Check sheet for the drawn part. Datum: minimum x, y, z corner. Units: mm. Coordinates: 2 decimals unless noted, no trailing zeros. Order: outer loops, then holes, each group sorted by start corner. A loop starts at its lowest first (then second) coordinate and runs counter-clockwise, first axis right, second up.
Q1. Thickness scan on line 1 (X direction, y = 3.75, z = 20); line 2 (Y direction, x = 27.5, z = 24.5). Record the ranges inside material, lowest first.
Q2. Cross-section at A-A, the plane z = 20. Record the boundary of the cut face in (x, y).
Q3. Cross-section at B-B, the plane x = 20. Record the boundary of the cut face in (y, z).
Q4. Depth check by flat-ended pin: P1, Ø1.5, axis at x = 23.5, z = 8.5, coming from the +Y side; P2, Ø2, axis at x = 33.5, y = 2, coming from the +Z side; P3, Ø1.5, axis at x = 15, y = 3.5, coming from the +Z side; P4, Ø1, axis at x = 12.5, z = 4, coming from the -Y side. Enter the tip coordinate at first touch or a pass-through.
Q5. Draft check along Z on the marked faces 1, 2 and 3. Enter one of: pulls with the +Z half, pulls with the -Z half, needs draft (parallel to the pull), parting line crosses it, or undercut.
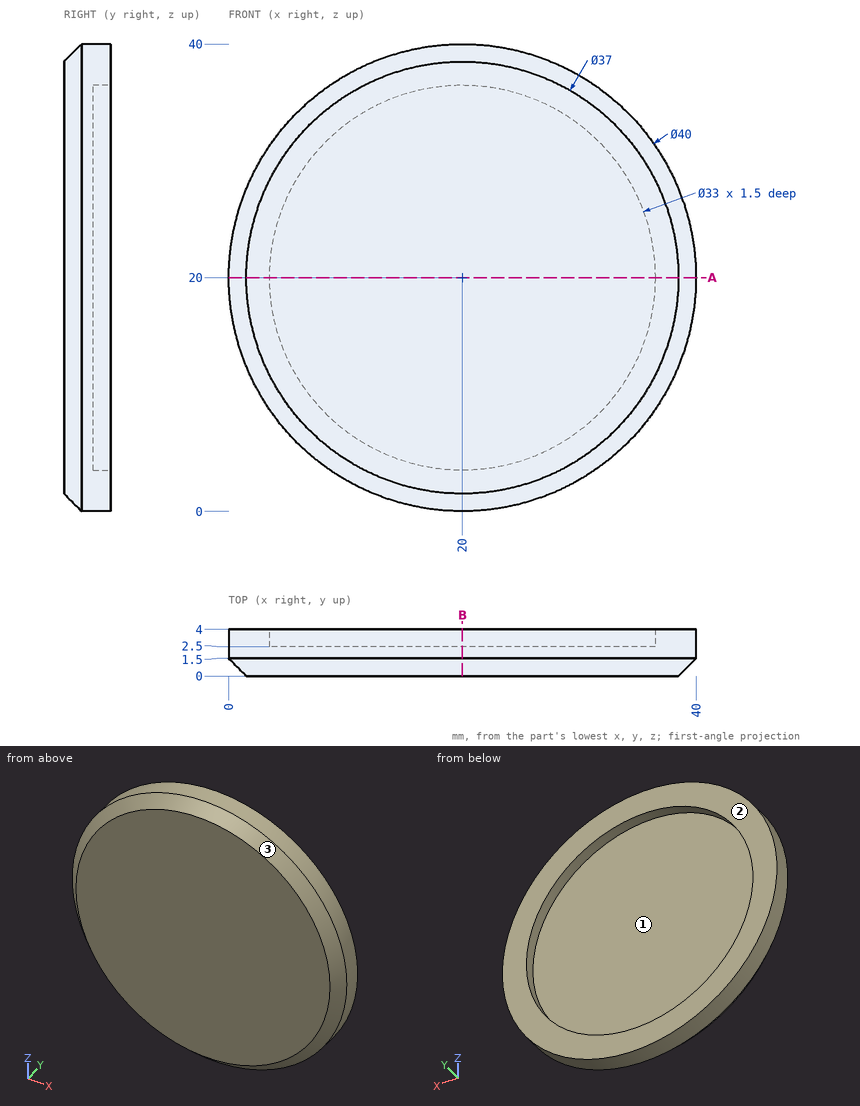
Check values:
1. line 1: x = 0 to 3.5, 36.5 to 40
1. line 2: y = 0 to 2.5
2. outline: (0, 1.5) - (1.5, 0) - (38.5, 0) - (40, 1.5) - (40, 4) - (36.5, 4) - (36.5, 2.5) - (3.5, 2.5) - (3.5, 4) - (0, 4) - close
3. outline: (0, 1.5) - (1.5, 0) - (4, 0) - (4, 3.5) - (2.5, 3.5) - (2.5, 36.5) - (4, 36.5) - (4, 40) - (1.5, 40) - (0, 38.5) - close
4. P1: stops at y = 2.5
4. P2: stops at z = 35.61
4. P3: stops at z = 39.54
4. P4: stops at y = 0
5. face 1: undercut
5. face 2: needs draft
5. face 3: parting line crosses it
